Study the drawing (mm; zero at the part's minimum x, y, z) and answer. Give positions to 0.01 mm unless a question says otherwise; leave off trailing zeros. Write each loop counter-clockwise with the first axis right and the second up, starting at its lowest first coordinate (ties: lowest second). Pieces come first, ordered by that corner, then holes. Notation, with made-up numbers: (-38.5, 37.25) - (20.5, 37.25) arc R23 cw to (20.5, 71.25) - close; hole circle Ø10 at (68, 59). An arc over 180 degrees is marked (long way). One line per item, written item: value. Start each with the question number.
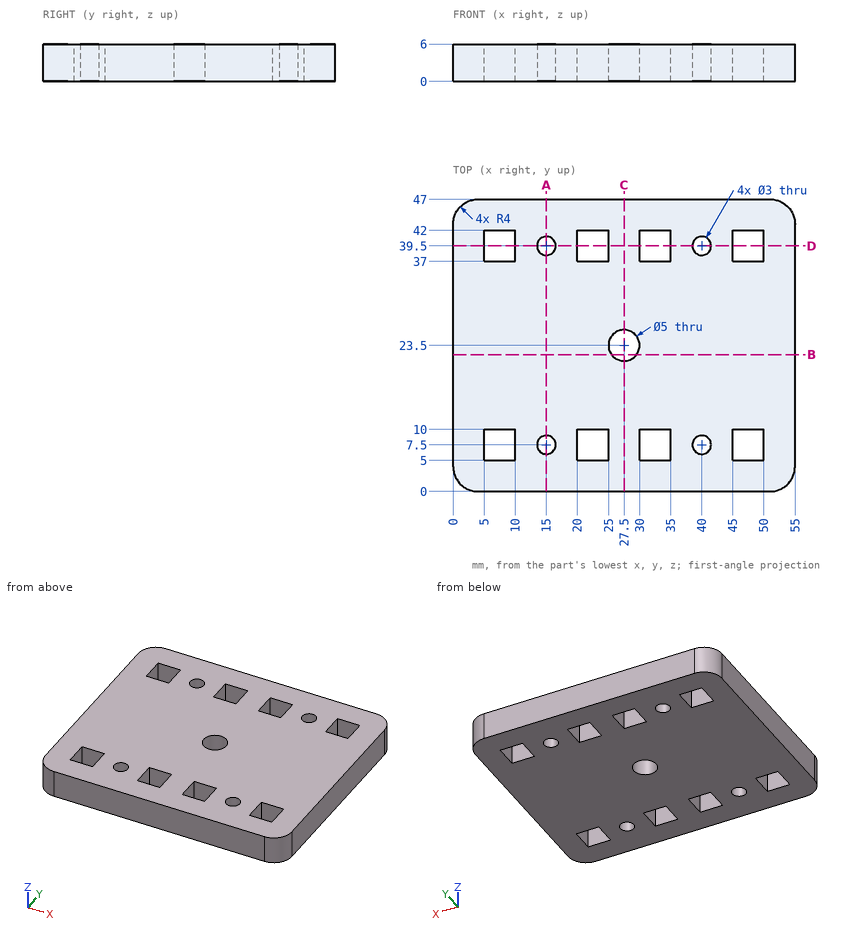
Item 1: Find section D-D on y = 39.5. Determine the outline of the cut face in (x, z), plus the area to 3 significant figures.
Item 2: Find section A-A on x = 15. Determine the outline of the cut face in (y, z).
Item 3: Each of these flat-tipped pins is pushed along its axis until it touches: pin 1 Ø2.5 at (x, y) = (15, 7.5) entering from +Z; pin 2 Ø3 at (x, z) = (37, 1) entering from -Y. Where does it stop, or does it pass through?
Item 4: Find section B-B on y = 22. Determine the outline of the cut face in (x, z), plus the area to 3 significant figures.
Item 5: Find section C-C on x = 27.5. Determine the outline of the cut face in (y, z).
Item 6: Straight lines are drawn through the part: line 1 along Y through (x, z) = (34.5, 0.5); line 2 along Y through (x, z) = (40, 2.6); line 3 along X through (y, z) = (41.5, 1.2). For each, find the intervals that lie inside material, in ascending order.
Values:
1. outline: (0, 0) - (5, 0) - (5, 6) - (0, 6) - close; (10, 0) - (13.5, 0) - (13.5, 6) - (10, 6) - close; (16.5, 0) - (20, 0) - (20, 6) - (16.5, 6) - close; (25, 0) - (30, 0) - (30, 6) - (25, 6) - close; (35, 0) - (38.5, 0) - (38.5, 6) - (35, 6) - close; (41.5, 0) - (45, 0) - (45, 6) - (41.5, 6) - close; (50, 0) - (55, 0) - (55, 6) - (50, 6) - close
1. area: 174 mm^2
2. outline: (0, 0) - (6, 0) - (6, 6) - (0, 6) - close; (9, 0) - (38, 0) - (38, 6) - (9, 6) - close; (41, 0) - (47, 0) - (47, 6) - (41, 6) - close
3. pin 1: through
3. pin 2: y = 0
4. outline: (0, 0) - (25.5, 0) - (25.5, 6) - (0, 6) - close; (29.5, 0) - (55, 0) - (55, 6) - (29.5, 6) - close
4. area: 306 mm^2
5. outline: (0, 0) - (21, 0) - (21, 6) - (0, 6) - close; (26, 0) - (47, 0) - (47, 6) - (26, 6) - close
6. line 1: 0 to 5, 10 to 37, 42 to 47
6. line 2: 0 to 6, 9 to 38, 41 to 47
6. line 3: 0 to 5, 10 to 20, 25 to 30, 35 to 45, 50 to 55
